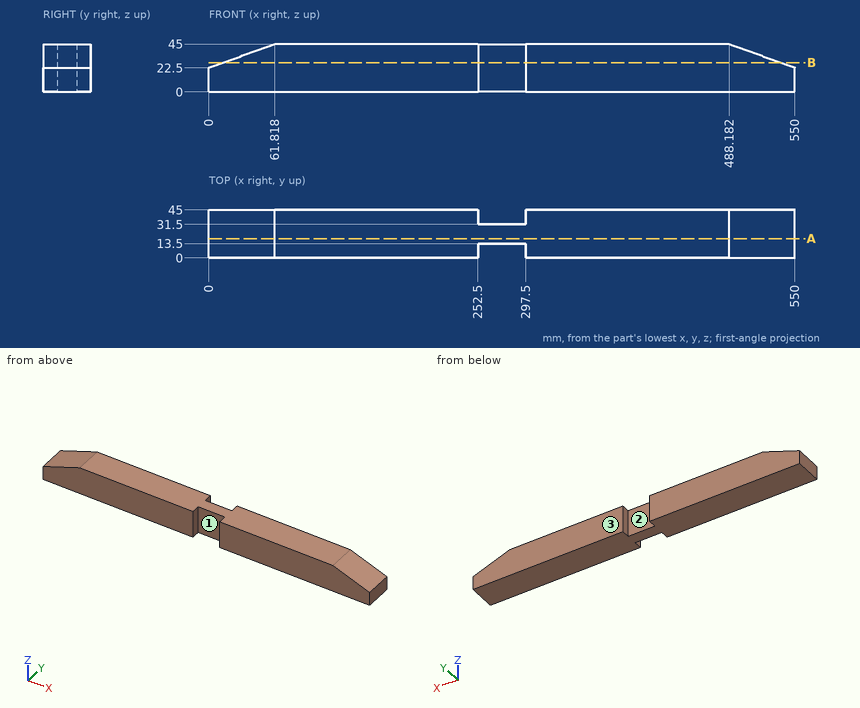
Could you check a few things on this drawing? It's one solid part, dimensions in mm from its lowest x, y, z. A direction names the side the tool comes from. Coordinates: 2 decimals unless noted, no trailing zeros. Order: outer loops, then holes, each group sorted by start corner. A loop starts at its lowest first (then second) coordinate and runs counter-clockwise, first axis right, second up. Notation, with made-up numbers: (-21.75, 71.5) -> (28.25, 71.5) arc R8 ccw to (28.25, 83.5) -> close; hole circle Ø8 at (19, 20.5). An arc over 180 degrees is marked (long way). One line per item, written item: value. Start each with the question number.
1) Imagine slicing it at A-A on y = 18. List the corners of the cut face in (x, z) for me.
2) Which directions (+Z, -Z, +X, -X, +Y, -Y) give clear straight access to the entire face, cutting with the end or side of a thin tool? Please do the marked faces 1, 2 and 3.
3) I'm going to push a flat-ended pin straight in: pin 1 (13.5 mm diameter, centred on x = 270.5, z = 19, fed in from -Y). Where does the tip first touch, or does it pass through?
4) Imagine slicing it at B-B on z = 27.5. List the corners of the cut face in (x, y) for me, plus the area to 3 significant figures.
5) If I drill on L1, parallel to X at y = 42, z = 20; L2, parallel to Y at x = 282.5, z = 19.5; L3, parallel to Z at x = 497, y = 7, over which ranges is the centre line in solid material (lowest first)? Write a range as [from, to].
Answer list:
1. outline: (0, 0) -> (550, 0) -> (550, 22.5) -> (488.18, 45) -> (61.82, 45) -> (0, 22.5) -> close
2. face 1: +Z, -Z, -Y
2. face 2: +Z, -Z, +Y
2. face 3: +Z, -Z, +X, -X, +Y
3. pin 1: stops at y = 13.5
4. outline: (13.74, 0) -> (252.5, 0) -> (252.5, 13.5) -> (297.5, 13.5) -> (297.5, 0) -> (536.26, 0) -> (536.26, 45) -> (297.5, 45) -> (297.5, 31.5) -> (252.5, 31.5) -> (252.5, 45) -> (13.74, 45) -> close
4. area: 22,300 mm2
5. L1: x = [0, 252.5], [297.5, 550]
5. L2: y = [13.5, 31.5]
5. L3: z = [0, 41.79]
